For this review, take the finished solid that the model builds, in its own axes (mm). Face numbers are marked on the shaded views. Round coordinates to 2 decimals unless told otherwise and drop trailing zeros. Write each loop counter-clockwise with the first axis right and the second up, starting at its lowest first coordinate (ties: lowest second). Pieces come first, ordered by that corner, then holes. Notation, with made-up numbers: (22.5, 58.25) -> (75.5, 58.25) arc R17 cw to (75.5, 67.25) -> close; hole circle Ø1 at (-23.5, 42.5). An arc over 180 degrees is marked (long way). Write each question's results on one line, items separated by ' | '. Start each with the question number.
Item 1: Add section A-A (y = -1.5). State the section outline as (x, z) points.
Item 2: Clearance check with flat-ended pins moving along their axes: pin 1 (1.5 mm diameter, centred on x = 15.5, y = -4, fed in from -Z); pin 2 (0.9 mm diameter, centred on y = -4, z = 5, fed in from +X); pin 3 (2.5 mm diameter, centred on x = -25, y = -4.5, fed in from +Z). State where each tip first meets the part, or that it passes through.
Item 3: Add section C-C (z = 0). State the section outline as (x, y) points, plus the area to 3 significant figures.
Item 4: To check wall thickness, follow line 1 along X through (y, z) = (-2.7, 0); line 2 along Z through (x, y) = (0, -3.15); line 3 along Z through (x, y) = (-9.5, -4.7). State the ranges of each line that lie inside material, in increasing order.
Item 5: The part is to be moulded in two halves that separate along X. For the marked faces 1 and 2, say which applies: +X half, -X half, draft (parallel to the pull), parting line (faces both ways), or undercut.
Item 6: Add section D-D (z = -15). State the section outline as (x, y) points.
Item 7: Add section B-B (x = 0). State the section outline as (y, z) points.
from build123d import *

# Parameters (mm, degrees)
SKETCH_W          = 55
SKETCH_H          = 38
PAD_DEPTH         = 3
SKETCH001_W       = 50.5
SKETCH001_H       = 33
PAD001_DEPTH      = 3
SKETCH003_R       = 1.75
SKETCH003_R_2     = 12
POCKET_DEPTH      = 5
POCKET_DEPTH_BACK = 5


with BuildPart() as part:
    # Sketch → Pad (new body)
    with BuildSketch(Plane.XZ):
        with Locations((27.5, 0)):
            Rectangle(SKETCH_W, SKETCH_H)
    pad = extrude(amount=PAD_DEPTH)

    # Sketch001 (on Face6 of Pad) → Pad001 (join)
    with BuildSketch(Plane.XZ.offset(3)):
        with Locations((25.25, -0.5)):
            Rectangle(SKETCH001_W, SKETCH001_H)
    pad001 = extrude(amount=PAD001_DEPTH)

    # Mirrored: Pad, Pad001 across Sketch V_Axis
    add(pad.mirror(Plane(origin=(0, 0, 0), x_dir=(0, -1, 0), z_dir=(1, 0, 0))))
    add(pad001.mirror(Plane(origin=(0, 0, 0), x_dir=(0, -1, 0), z_dir=(1, 0, 0))))

    # Sketch003 → Pocket (cut, two sides)
    with BuildSketch(Plane(origin=(0, -3, 0), x_dir=(1, 0, 0), z_dir=(0, 1, 0))) as pocket_sk:
        with Locations((9.5, -12)):
            Circle(SKETCH003_R)
        with Locations((-9.5, 12)):
            Circle(SKETCH003_R)
        Circle(SKETCH003_R_2)
    extrude(amount=POCKET_DEPTH, mode=Mode.SUBTRACT)
    extrude(pocket_sk.sketch, amount=-POCKET_DEPTH_BACK, mode=Mode.SUBTRACT)


solid = part.part
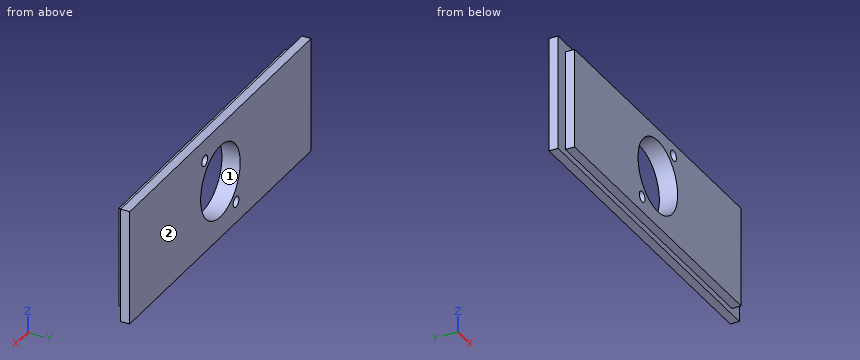
Responses:
1) outline: (-55, -19) -> (55, -19) -> (55, 19) -> (-55, 19) -> close; hole circle Ø24 at (0, 0); hole circle Ø3.5 at (-9.5, -12); hole circle Ø3.5 at (9.5, 12)
2) pin 1: stops at z = -17 | pin 2: stops at x = 50.5 | pin 3: stops at z = 16
3) outline: (-55, -3) -> (-50.5, -3) -> (-50.5, -6) -> (-12, -6) -> (-12, 0) -> (-55, 0) -> close; (12, -6) -> (50.5, -6) -> (50.5, -3) -> (55, -3) -> (55, 0) -> (12, 0) -> close | area: 489 mm^2
4) line 1: x = -55 to -12, 12 to 55 | line 2: z = -17 to -12, 12 to 16 | line 3: z = -17 to -13.75, -10.25 to -7.33, 7.33 to 16
5) face 1: undercut | face 2: draft
6) outline: (-55, -3) -> (-50.5, -3) -> (-50.5, -6) -> (50.5, -6) -> (50.5, -3) -> (55, -3) -> (55, 0) -> (-55, 0) -> close
7) outline: (-6, -17) -> (-3, -17) -> (-3, -19) -> (0, -19) -> (0, -12) -> (-6, -12) -> close; (-6, 12) -> (0, 12) -> (0, 19) -> (-3, 19) -> (-3, 16) -> (-6, 16) -> close
